Geometry: final body of the model. Coordinates: model frame, mm. Face numbers are marked on the shaded views. A direction names the side the tool comes from. Give positions to 0.01 mm unless a question says otherwise; leave off trailing zeros. Order: outer loops, then holes, each group sorted by start corner. A loop starts at its lowest first (then second) coordinate and runs counter-clockwise, first axis right, second up. Notation, with made-up numbers: (71, -33) - (106, -33) arc R23 cw to (106, 1) - close; hole circle Ø8 at (-32, 83). An arc over 180 degrees is marked (long way). One line per item, written item: value.
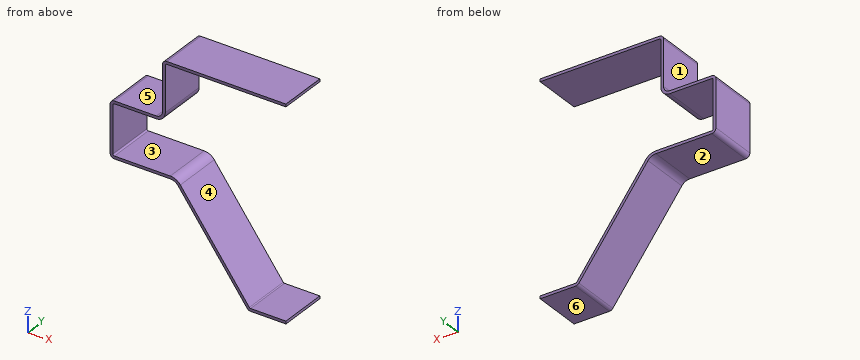
Autodesk Inventor part; units mm, degrees
ref_plane "YZ Plane" through (0, 0, 0) normal (1, 0, 0) x (0, 1, 0)
ref_plane "XZ Plane" through (0, 0, 0) normal (0, 1, 0) x (-1, 0, 0)
ref_plane "XY Plane" through (0, 0, 0) normal (0, 0, 1) x (1, 0, 0)
sketch "Boceto1" plane through (0, 0, 0) normal (0, 1, 0) x (-1, 0, 0)
  line L0 (0, 0) -> (273.05, 0)
  line L1 (273.05, 0) -> (273.05, -101.6)
  line L2 (273.05, -101.6) -> (368.3, -101.6)
  line L3 (368.3, -101.6) -> (368.3, -212.725)
  line L4 (0, 0) -> (0, -393.7)
  line L5 (0, -393.7) -> (114.3, -393.7)
  line L6 (368.3, -212.725) -> (247.65, -212.725)
  line L7 (247.65, -212.725) -> (114.3, -393.7)
  dimension "d0" = 273.05
  dimension "d1" = 101.6
  dimension "d2" = 95.25
  dimension "d3" = 111.125
  dimension "d4" = 393.7
  dimension "d50" = 114.3
  dimension "d51" = 133.35
extrude "Extrusión1" add sketch "Boceto1" along normal blind 5
fillet "Empalme1" radius 12.7 7 edges at (-368.3, 2.5, -101.6) (-273.05, 2.5, 0) (-368.3, 2.5, -212.725) (-247.65, 2.5, -212.725) (-114.3, 2.5, -393.7) (0, 2.5, -393.7) (0, 2.5, 0)
fillet "Empalme2" radius 6.35 1 edges at (-273.05, 2.5, -101.6)
sketch "Boceto2" plane through (0, 5, 0) normal (0, 1, 0) x (1, 0, 0)
  line L0 (-349.25, 119.0625) -> (-273.05, 119.0625)
  line L1 (-273.05, 119.0625) -> (-273.05, 195.2625)
  line L2 (-273.05, 195.2625) -> (-349.25, 195.2625)
  line L3 (-349.25, 195.2625) -> (-349.25, 119.0625)
  line L4 (-368.3, 200.025) -> (-368.3, 114.3)
  line L5 (-254.0674, 212.725) -> (-355.6, 212.725)
  line L6 (-355.6, 101.6) -> (-279.4, 101.6)
  line L7 (-260.35, 0) -> (-12.7, 0)
  line L8 (-43.6563, 0) -> (-38.1, 0)
  line L9 (-38.1, 0) -> (-38.1, 6.35)
  line L10 (-38.1, 6.35) -> (-43.6562, 6.35)
  line L11 (-43.6562, 6.35) -> (-43.6563, 0)
  line L12 (-12.7, 393.7) -> (-107.8826, 393.7)
  line L13 (0, 12.7) -> (0, 381)
  circle A0 centre (-98.0281, 104.775) radius 4.3656
  circle A1 centre (-59.9281, 104.775) radius 4.3656
  circle A2 centre (-98.0281, 288.925) radius 4.3656
  circle A3 centre (-59.9281, 288.925) radius 4.3656
  line L14 (-123.825, 158.75) -> (-47.625, 158.75)
  line L15 (-47.625, 158.75) -> (-47.625, 234.95)
  line L16 (-47.625, 234.95) -> (-123.825, 234.95)
  line L17 (-123.825, 234.95) -> (-123.825, 158.75)
  circle A4 centre (-42.6641, 365.125) radius 5
  circle A5 centre (-42.6641, 28.575) radius 5
  line L18 (-107.8826, 393.7) -> (-12.7, 393.7)
  line L19 (-43.6563, 393.7) -> (-38.1, 393.7)
  line L20 (-38.1, 393.7) -> (-38.1, 387.35)
  line L21 (-38.1, 387.35) -> (-43.6563, 387.35)
  line L22 (-43.6563, 387.35) -> (-43.6563, 393.7)
  line L23 (-42.8625, 127) -> (-38.1, 127)
  line L24 (-38.1, 127) -> (-38.1, 140.0969)
  line L25 (-38.1, 140.0969) -> (-42.8625, 140.0969)
  line L26 (-42.8625, 140.0969) -> (-42.8625, 127)
  line L27 (-42.8625, 190.5) -> (-38.1, 190.5)
  line L28 (-38.1, 190.5) -> (-38.1, 203.5969)
  line L29 (-38.1, 203.5969) -> (-42.8625, 203.5969)
  line L30 (-42.8625, 203.5969) -> (-42.8625, 190.5)
  line L31 (-42.8625, 254) -> (-38.1, 254)
  line L32 (-38.1, 254) -> (-38.1, 267.0969)
  line L33 (-38.1, 267.0969) -> (-42.8625, 267.0969)
  line L34 (-42.8625, 267.0969) -> (-42.8625, 254)
  point P0 (0, 0)
  dimension "d11" = 76.2
  dimension "d17" = 17.4625
  dimension "d18" = 19.05
  dimension "d19" = 76.2
  dimension "d20" = 5.5563
  dimension "d22" = 6.35
  dimension "d24" = 38.1
  dimension "d27" = 8.7312
  dimension "d38" = 76.2
  dimension "d39" = 76.2
  dimension "d40" = 158.75
  dimension "d42" = 10
  dimension "d43" = 28.575
  dimension "d44" = 42.6641
  dimension "d47" = 10
  dimension "d52" = 38.1
  dimension "d53" = 5.5563
  dimension "d54" = 6.35
  dimension "d55" = 47.625
  dimension "d56" = 8.7312
  dimension "d57" = 98.0281
  dimension "d58" = 38.1
  dimension "d59" = 53.975
  dimension "d60" = 53.975
  dimension "d61" = 184.15
  dimension "d62" = 184.15
  dimension "d63" = 38.1
  dimension "d64" = 8.7312
  dimension "d65" = 8.7312
  dimension "d66" = 98.0281
  dimension "d67" = 42.6641
  dimension "d68" = 28.575
  dimension "d69" = 4.7625
  dimension "d70" = 4.7625
  dimension "d71" = 4.7625
  dimension "d72" = 13.0969
  dimension "d73" = 13.0969
  dimension "d74" = 13.0969
  dimension "d75" = 38.1
  dimension "d80" = 63.5
  dimension "d81" = 63.5
  dimension "d82" = 127
extrude "Extrusión2" cut sketch "Boceto2" against normal up to next
fillet "Empalme3" radius 3.5719 8 edges at (-349.25, 2.5, -119.0625) (-123.825, 2.5, -158.75) (-349.25, 2.5, -195.2625) (-123.825, 2.5, -234.95) (-273.05, 2.5, -195.2625) (-47.625, 2.5, -234.95) (-273.05, 2.5, -119.0625) (-47.625, 2.5, -158.75)
sketch "Boceto3" plane through (0, 5, 0) normal (0, 1, 0) x (1, 0, 0)
  line L0 (0, 12.7) -> (0, 381)
  line L1 (0, 381) -> (0, 12.7)
  line L2 (0, 196.85) -> (-12.7, 196.85)
  line L3 (0, 196.85) -> (0, 219.075)
  line L4 (0, 196.85) -> (0, 174.625)
  arc A0 (0, 219.075) -> (0, 174.625) centre (13.0969, 196.85) ccw
  point P0 (0, 0)
  dimension "d86" = 12.7
  dimension "d87" = 22.225
  dimension "d88" = 22.225
extrude "Extrusión3" cut sketch "Boceto3" against normal up to next
fillet "Empalme4" radius 4.7625 2 edges at (0, 2.5, -219.075) (0, 2.5, -174.625)
sketch "Boceto4" plane through (0, 0, 0) normal (0, -1, 0) x (1, 0, 0)
  line L0 (-43.6562, -5) -> (-260.35, -5)
  line L1 (-268.05, -12.7) -> (-268.05, -95.25)
  line L2 (-279.4, -106.6) -> (-355.6, -106.6)
  line L3 (-363.3, -114.3) -> (-363.3, -200.025)
  line L4 (-355.6, -207.725) -> (-254.0138, -207.725)
  line L5 (-239.693, -214.9673) -> (-114.1714, -385.5509)
  line L6 (-107.9443, -388.7) -> (-43.6563, -388.7)
  line L7 (-107.8826, -393.7) -> (-43.6563, -393.7)
  line L8 (-118.1068, -388.5336) -> (-243.8432, -217.8914)
  line L9 (-355.6, -212.725) -> (-254.0674, -212.725)
  line L10 (-368.3, -200.025) -> (-368.3, -114.3)
  line L11 (-43.6563, -387.35) -> (-43.6563, -393.7)
  line L12 (-355.6, -101.6) -> (-279.4, -101.6)
  line L13 (-273.05, -95.25) -> (-273.05, -12.7)
  line L14 (-260.35, 0) -> (-43.6563, 0)
  line L15 (-43.6563, 0) -> (-43.6562, -6.35)
  arc A0 (-363.3, -200.025) -> (-355.6, -207.725) centre (-355.6, -200.025) ccw
  line L16 (-368.3, -114.3) -> (-368.3, -200.025)
  arc A1 (-355.6, -106.6) -> (-363.3, -114.3) centre (-355.6, -114.3) ccw
  arc A2 (-260.35, -5) -> (-268.05, -12.7) centre (-260.35, -12.7) ccw
  arc A3 (-279.4, -106.6) -> (-268.05, -95.25) centre (-279.4, -95.25) ccw
  line L17 (-273.05, -12.7) -> (-273.05, -95.25)
  line L18 (-174.9103, -311.4431) -> (-170.8831, -308.4798)
  arc A4 (-239.693, -214.9673) -> (-254.0138, -207.725) centre (-254.0138, -225.505) ccw
  arc A5 (-114.1714, -385.5509) -> (-107.9443, -388.7) centre (-107.9443, -380.9688) ccw
  line L19 (-43.6563, -383.7) -> (-107.9443, -383.7)
  arc A6 (-110.1442, -382.5875) -> (-107.9443, -383.7) centre (-107.9443, -380.9688) ccw
  line L20 (-110.1442, -382.5875) -> (-235.6658, -212.0039)
  arc A7 (-235.6658, -212.0039) -> (-254.0138, -202.725) centre (-254.0138, -225.505) ccw
  line L21 (-254.0138, -202.725) -> (-355.6, -202.725)
  arc A8 (-358.3, -200.025) -> (-355.6, -202.725) centre (-355.6, -200.025) ccw
  line L22 (-358.3, -200.025) -> (-358.3, -114.3)
  arc A9 (-355.6, -111.6) -> (-358.3, -114.3) centre (-355.6, -114.3) ccw
  line L23 (-355.6, -111.6) -> (-279.4, -111.6)
  arc A10 (-279.4, -111.6) -> (-263.05, -95.25) centre (-279.4, -95.25) ccw
  line L24 (-263.05, -95.25) -> (-263.05, -12.7)
  arc A11 (-260.35, -10) -> (-263.05, -12.7) centre (-260.35, -12.7) ccw
  line L25 (-260.35, -10) -> (-43.6562, -10)
  line L26 (-43.6563, -383.7) -> (-43.6563, -388.7)
  line L27 (-43.6562, -5) -> (-43.6562, -10)
  line L28 (-43.6562, -6.35) -> (-43.6563, 0)
  point P0 (0, 0)
  dimension "d92" = 5
  dimension "d95" = 5
  dimension "d96" = 5
  dimension "d99" = 5
  dimension "d100" = 5
  dimension "d101" = 5
  dimension "d102" = 0
  dimension "d105" = 0
  dimension "d109" = 0
  dimension "d110" = 5
  dimension "d115" = 17.78
  dimension "d117" = 5
  dimension "d118" = 7.7312
extrude "Extrusión4" add sketch "Boceto4" along normal blind 88.9
sketch "Boceto5" plane through (0, 5, 0) normal (0, 1, 0) x (1, 0, 0)
  line L0 (88.3096, -76.4471) -> (-485.0439, -76.4471)
  line L1 (-485.0439, -76.4471) -> (-485.0439, 517.9952)
  line L2 (-485.0439, 517.9952) -> (88.3096, 517.9952)
  line L3 (88.3096, 517.9952) -> (88.3096, -76.4471)
  point P0 (0, 0)
extrude "Extrusión5" cut sketch "Boceto5" against normal up to surface (5 mm away)
equation "\"d42\" = UBD"
equation "\"d47\" = UBD"
equation "\"LM\" = 76.2"
equation "\"UBD\" = 10"
properties part number "CAR INTERNAL PLATE"
1) Material intervals for line 1 along Z through (x, y) = (-299.5, -70) (3 decimals); line 2 along Z through (x, y) = (-93.5, -20.5); line 3 along X through (y, z) = (-14, -180), sorted ascending.
Answers below:
line 1: -207.725 to -202.725, -111.6 to -106.6
line 2: -388.7 to -383.7, -10 to -5
line 3: -363.3 to -358.3
2) Set-up query: the marked faces 1, 2 and 3. Return all of +Z, -Z, +X, -X, +Y, -Y with unobstructed straight access to the full face (end or side cutting, diameter ignored); none if empty.
Answers below:
face 1: +Z, -X, +Y, -Y
face 2: -Z, -X, +Y, -Y
face 3: +X, +Y, -Y
3) First-contact query: pin 1 (5 mm diameter, centred on y = -59.5, z = -293.5, fed in from -X); pin 2 (1 mm diameter, centred on y = -32.5, z = -336.5, fed in from -X); pin 3 (1.5 mm diameter, centred on x = -174, y = -27.5, fed in from -Z). Flat tips, straight axial feed; report the tip coordinate or a pass-through.
Answers below:
pin 1: x = -183.75
pin 2: x = -150.63
pin 3: z = -305.26
4) Section C-C, the plane z = -159.5. Return loops of the section in (x, y), then the cut area to 4 significant figures.
Answers below:
outline: (-363.3, -88.9) - (-358.3, -88.9) - (-358.3, 0) - (-363.3, 0) - close
area: 444.5 mm^2
5) Section A-A, the plane x = -289. Return loops of the section in (y, z) (3 decimals), then the cut area to 3 significant figures.
Answers below:
outline: (-88.9, -207.725) - (0, -207.725) - (0, -202.725) - (-88.9, -202.725) - close; (-88.9, -111.6) - (0, -111.6) - (0, -106.6) - (-88.9, -106.6) - close
area: 889 mm^2
6) Mould query, pull axis Z, two halves, no side actions, for the marked faces 4, 5 and 6. Classes: released by +Z, released by -Z, zero draft, split by the parting line, or undercut.
Answers below:
face 4: undercut
face 5: released by +Z
face 6: released by -Z
7) Section D-D, the plane x = -129. Return loops of the section in (y, z).
Answers below:
outline: (-88.9, -365.4) - (0, -365.4) - (0, -356.96) - (-88.9, -356.96) - close; (-88.9, -10) - (0, -10) - (0, -5) - (-88.9, -5) - close
